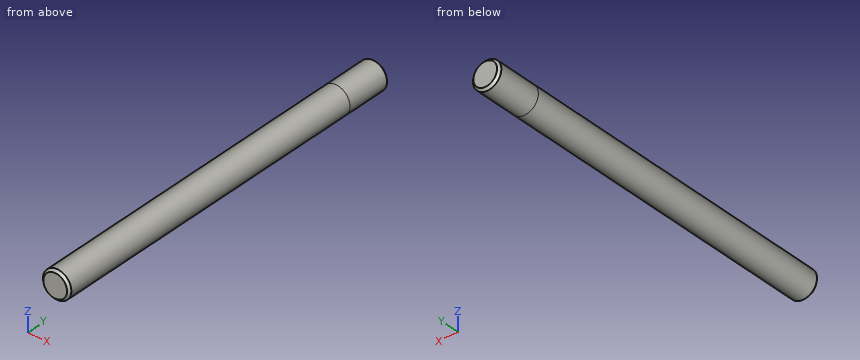
Autodesk Inventor part; units mm, degrees
ref_plane "YZ Plane" through (0, 0, 0) normal (1, 0, 0) x (0, 1, 0)
ref_plane "XZ Plane" through (0, 0, 0) normal (0, 1, 0) x (-1, 0, 0)
ref_plane "XY Plane" through (0, 0, 0) normal (0, 0, 1) x (1, 0, 0)
sketch "Sketch1" plane through (0, 0, 0) normal (0, 1, 0) x (-1, 0, 0)
  circle A0 centre (0, 0) radius 3
  dimension "d3" = 6
extrude "Extrusion2" add sketch "Sketch1" along normal blind 10
thread "Thread1"
sketch "Sketch3" plane through (0, 10, 0) normal (0, 1, 0) x (1, 0, 0)
  circle A0 centre (0, 0) radius 3
  dimension "d8" = 6
extrude "Extrusion3" add sketch "Sketch3" along normal blind 62
sketch "Sketch4" plane through (0, 72, 0) normal (0, 1, 0) x (1, 0, 0)
  circle A0 centre (0, 0) radius 3
  circle A1 centre (0, 0) radius 3
  dimension "d11" = 6
extrude "Extrusion4" add sketch "Sketch4" along normal blind 10
thread "Thread2"
chamfer "Chamfer1" distance 0.5 distance2 0.5 1 edges at (-3, 82, 0) measured on face at (-0.5351, 82, -1.0949)
chamfer "Chamfer2" distance 0.5 distance2 0.5 1 edges at (3, 0, 0) measured on face at (0.5351, 0, 1.0949)
properties part number "cylinder head bolt"
CAD build for the part. Positions are in the model's coordinates, mm. Coordinates: 2 decimals unless noted, no trailing zeros. Loops run counter-clockwise (first coordinate to the right, second up) from the corner with the lowest first, then second, coordinate; pieces in that order, holes last. Notation, with made-up numbers: (57, -36.5) - (105, -36.5) arc R21 ccw to (105, 0.5) - close; hole circle Ø8 at (-23, 15.5). An arc over 180 degrees is marked (long way). Write item = value, one per line. Start each with the question number.
Q1. Flat gauge pins, fed straight in: pin 1 Ø1 at (y, z) = (19, 1.5) entering from -X; pin 2 Ø1.5 at (x, y) = (2, 45) entering from -Z; pin 3 Ø1 at (x, y) = (1, 66) entering from -Z. Where does each tip first touch, or does it go through?
Q2. Drill centre lines: L1, parallel to Z at x = 0.2, y = 64.5; L2, parallel to X at y = 60.5, z = 2.6; L3, parallel to X at y = 50.5, z = 2.3. Where is each one in solid material? Low to high.
Q3. Cut at A-A, the plane y = 11.5. List the corners of the cut face in (x, z).
Computed:
q1.pin_1 = -2.83
q1.pin_2 = -2.73
q1.pin_3 = -2.96
q2.L1 = -2.99 to 2.99
q2.L2 = -1.5 to 1.5
q2.L3 = -1.93 to 1.93
q3.outline = circle Ø6 at (0, 0)
